Design review of the part built by this model. Coordinates are the model's own, in mm. Give positions to 0.01 mm unless a question says otherwise; leave off trailing zeros. Use CSV: the item, a comma, the result in double quotes.
```python
from build123d import *

# Parameters (mm, degrees)
SKETCH1_R               = 2.5
EXTRUDE1_DEPTH          = 510
CUT_EXTRUDE1_DEPTH      = 511.979451642
CUT_EXTRUDE1_DEPTH_BACK = 511.979451642
SKETCH2_W               = 3.3
SKETCH2_H               = 11.078679656


with BuildPart() as part:
    # Sketch1 → Extrude1 (new body)
    with BuildSketch(Plane.XY):
        with BuildLine():
            Line((0, 3.9), (-2.010912703, 3.9))
            ThreePointArc((-2.010912703, 3.9), (-2.776279568, 4.052240935), (-3.425126266, 4.485786438))
            Line((-3.425126266, 4.485786438), (-5.539339828, 6.6))
            Line((-5.539339828, 6.6), (-5.539339828, 8.2))
            Line((-5.539339828, 8.2), (-3.1, 8.2))
            Line((-3.1, 8.2), (-3.1, 9.5))
            Line((-3.1, 9.5), (-3.4, 9.5))
            ThreePointArc((-3.4, 9.5), (-3.541421356, 9.558578644), (-3.6, 9.7))
            Line((-3.6, 9.7), (-3.6, 10))
            Line((-3.6, 10), (-8.5, 10))
            Line((-8.5, 10), (-11.5, 10))
            Line((-11.5, 10), (-16.4, 10))
            Line((-16.4, 10), (-16.4, 9.7))
            ThreePointArc((-16.4, 9.7), (-16.458578644, 9.558578644), (-16.6, 9.5))
            Line((-16.6, 9.5), (-16.9, 9.5))
            Line((-16.9, 9.5), (-16.9, 8.2))
            Line((-16.9, 8.2), (-14.460660172, 8.2))
            Line((-14.460660172, 8.2), (-14.460660172, 6.6))
            Line((-14.460660172, 6.6), (-16.574873734, 4.485786438))
            ThreePointArc((-16.574873734, 4.485786438), (-17.223720432, 4.052240935), (-17.989087297, 3.9))
            Line((-17.989087297, 3.9), (-20, 3.9))
            Line((-20, 3.9), (-22.010912703, 3.9))
            ThreePointArc((-22.010912703, 3.9), (-22.776279568, 4.052240935), (-23.425126266, 4.485786438))
            Line((-23.425126266, 4.485786438), (-25.539339828, 6.6))
            Line((-25.539339828, 6.6), (-25.539339828, 8.2))
            Line((-25.539339828, 8.2), (-23.1, 8.2))
            Line((-23.1, 8.2), (-23.1, 9.5))
            Line((-23.1, 9.5), (-23.4, 9.5))
            ThreePointArc((-23.4, 9.5), (-23.541421356, 9.558578644), (-23.6, 9.7))
            Line((-23.6, 9.7), (-23.6, 10))
            Line((-23.6, 10), (-28.5, 10))
            ThreePointArc((-28.5, 10), (-29.560660172, 9.560660172), (-30, 8.5))
            Line((-30, 8.5), (-30, 3.6))
            Line((-30, 3.6), (-29.7, 3.6))
            ThreePointArc((-29.7, 3.6), (-29.558578644, 3.541421356), (-29.5, 3.4))
            Line((-29.5, 3.4), (-29.5, 3.1))
            Line((-29.5, 3.1), (-28.2, 3.1))
            Line((-28.2, 3.1), (-28.2, 5.539339828))
            Line((-28.2, 5.539339828), (-26.6, 5.539339828))
            Line((-26.6, 5.539339828), (-24.485786438, 3.425126266))
            ThreePointArc((-24.485786438, 3.425126266), (-24.052240935, 2.776279568), (-23.9, 2.010912703))
            Line((-23.9, 2.010912703), (-23.9, 0))
            Line((-23.9, 0), (-23.9, -2.010912703))
            ThreePointArc((-23.9, -2.010912703), (-24.052240935, -2.776279568), (-24.485786438, -3.425126266))
            Line((-24.485786438, -3.425126266), (-26.6, -5.539339828))
            Line((-26.6, -5.539339828), (-28.2, -5.539339828))
            Line((-28.2, -5.539339828), (-28.2, -3.1))
            Line((-28.2, -3.1), (-29.5, -3.1))
            Line((-29.5, -3.1), (-29.5, -3.4))
            ThreePointArc((-29.5, -3.4), (-29.558578644, -3.541421356), (-29.7, -3.6))
            Line((-29.7, -3.6), (-30, -3.6))
            Line((-30, -3.6), (-30, -8.5))
            ThreePointArc((-30, -8.5), (-29.560660172, -9.560660172), (-28.5, -10))
            Line((-28.5, -10), (-23.6, -10))
            Line((-23.6, -10), (-23.6, -9.7))
            ThreePointArc((-23.6, -9.7), (-23.541421356, -9.558578644), (-23.4, -9.5))
            Line((-23.4, -9.5), (-23.1, -9.5))
            Line((-23.1, -9.5), (-23.1, -8.2))
            Line((-23.1, -8.2), (-25.539339828, -8.2))
            Line((-25.539339828, -8.2), (-25.539339828, -6.6))
            Line((-25.539339828, -6.6), (-23.425126266, -4.485786438))
            ThreePointArc((-23.425126266, -4.485786438), (-22.776279568, -4.052240935), (-22.010912703, -3.9))
            Line((-22.010912703, -3.9), (-20, -3.9))
            Line((-20, -3.9), (-17.989087297, -3.9))
            ThreePointArc((-17.989087297, -3.9), (-17.223720432, -4.052240935), (-16.574873734, -4.485786438))
            Line((-16.574873734, -4.485786438), (-14.460660172, -6.6))
            Line((-14.460660172, -6.6), (-14.460660172, -8.2))
            Line((-14.460660172, -8.2), (-16.9, -8.2))
            Line((-16.9, -8.2), (-16.9, -9.5))
            Line((-16.9, -9.5), (-16.6, -9.5))
            ThreePointArc((-16.6, -9.5), (-16.458578644, -9.558578644), (-16.4, -9.7))
            Line((-16.4, -9.7), (-16.4, -10))
            Line((-16.4, -10), (-11.5, -10))
            Line((-11.5, -10), (-8.5, -10))
            Line((-8.5, -10), (-3.6, -10))
            Line((-3.6, -10), (-3.6, -9.7))
            ThreePointArc((-3.6, -9.7), (-3.541421356, -9.558578644), (-3.4, -9.5))
            Line((-3.4, -9.5), (-3.1, -9.5))
            Line((-3.1, -9.5), (-3.1, -8.2))
            Line((-3.1, -8.2), (-5.539339828, -8.2))
            Line((-5.539339828, -8.2), (-5.539339828, -6.6))
            Line((-5.539339828, -6.6), (-3.425126266, -4.485786438))
            ThreePointArc((-3.425126266, -4.485786438), (-2.776279568, -4.052240935), (-2.010912703, -3.9))
            Line((-2.010912703, -3.9), (0, -3.9))
            Line((0, -3.9), (2.010912703, -3.9))
            ThreePointArc((2.010912703, -3.9), (2.776279568, -4.052240935), (3.425126266, -4.485786438))
            Line((3.425126266, -4.485786438), (5.539339828, -6.6))
            Line((5.539339828, -6.6), (5.539339828, -8.2))
            Line((5.539339828, -8.2), (3.1, -8.2))
            Line((3.1, -8.2), (3.1, -9.5))
            Line((3.1, -9.5), (3.4, -9.5))
            ThreePointArc((3.4, -9.5), (3.541421356, -9.558578644), (3.6, -9.7))
            Line((3.6, -9.7), (3.6, -10))
            Line((3.6, -10), (8.5, -10))
            ThreePointArc((8.5, -10), (9.560660172, -9.560660172), (10, -8.5))
            Line((10, -8.5), (10, -3.6))
            Line((10, -3.6), (9.7, -3.6))
            ThreePointArc((9.7, -3.6), (9.558578644, -3.541421356), (9.5, -3.4))
            Line((9.5, -3.4), (9.5, -3.1))
            Line((9.5, -3.1), (8.2, -3.1))
            Line((8.2, -3.1), (8.2, -5.539339828))
            Line((8.2, -5.539339828), (6.6, -5.539339828))
            Line((6.6, -5.539339828), (4.485786438, -3.425126266))
            ThreePointArc((4.485786438, -3.425126266), (4.052240935, -2.776279568), (3.9, -2.010912703))
            Line((3.9, -2.010912703), (3.9, 0))
            Line((3.9, 0), (3.9, 2.010912703))
            ThreePointArc((3.9, 2.010912703), (4.052240935, 2.776279568), (4.485786438, 3.425126266))
            Line((4.485786438, 3.425126266), (6.6, 5.539339828))
            Line((6.6, 5.539339828), (8.2, 5.539339828))
            Line((8.2, 5.539339828), (8.2, 3.1))
            Line((8.2, 3.1), (9.5, 3.1))
            Line((9.5, 3.1), (9.5, 3.4))
            ThreePointArc((9.5, 3.4), (9.558578644, 3.541421356), (9.7, 3.6))
            Line((9.7, 3.6), (10, 3.6))
            Line((10, 3.6), (10, 8.5))
            ThreePointArc((10, 8.5), (9.560660172, 9.560660172), (8.5, 10))
            Line((8.5, 10), (3.6, 10))
            Line((3.6, 10), (3.6, 9.7))
            ThreePointArc((3.6, 9.7), (3.541421356, 9.558578644), (3.4, 9.5))
            Line((3.4, 9.5), (3.1, 9.5))
            Line((3.1, 9.5), (3.1, 8.2))
            Line((3.1, 8.2), (5.539339828, 8.2))
            Line((5.539339828, 8.2), (5.539339828, 6.6))
            Line((5.539339828, 6.6), (3.425126266, 4.485786438))
            ThreePointArc((3.425126266, 4.485786438), (2.776279568, 4.052240935), (2.010912703, 3.9))
            Line((2.010912703, 3.9), (0, 3.9))
        make_face()
        Circle(SKETCH1_R, mode=Mode.SUBTRACT)
        with Locations(Location((-20, 0, 0), (0, 0, 180))):
            Circle(SKETCH1_R, mode=Mode.SUBTRACT)
        with BuildLine():
            Line((-9.7, 3.6), (-10, 3.6))
            ThreePointArc((-10, 3.6), (-10.141421356, 3.541421356), (-10.2, 3.4))
            Line((-10.2, 3.4), (-10.2, 3.1))
            Line((-10.2, 3.1), (-11.5, 3.1))
            Line((-11.5, 3.1), (-11.5, 5.539339828))
            Line((-11.5, 5.539339828), (-13.1, 5.539339828))
            Line((-13.1, 5.539339828), (-15.214213562, 3.425126266))
            ThreePointArc((-15.214213562, 3.425126266), (-15.647759065, 2.776279568), (-15.8, 2.010912703))
            Line((-15.8, 2.010912703), (-15.8, 0))
            Line((-15.8, 0), (-15.8, -2.010912703))
            ThreePointArc((-15.8, -2.010912703), (-15.647759065, -2.776279568), (-15.214213562, -3.425126266))
            Line((-15.214213562, -3.425126266), (-13.1, -5.539339828))
            Line((-13.1, -5.539339828), (-11.5, -5.539339828))
            Line((-11.5, -5.539339828), (-11.5, -3.1))
            Line((-11.5, -3.1), (-10.2, -3.1))
            Line((-10.2, -3.1), (-10.2, -3.4))
            ThreePointArc((-10.2, -3.4), (-10.141421356, -3.541421356), (-10, -3.6))
            Line((-10, -3.6), (-9.7, -3.6))
            ThreePointArc((-9.7, -3.6), (-9.558578644, -3.541421356), (-9.5, -3.4))
            Line((-9.5, -3.4), (-9.5, -3.1))
            Line((-9.5, -3.1), (-8.2, -3.1))
            Line((-8.2, -3.1), (-8.2, -5.539339828))
            Line((-8.2, -5.539339828), (-6.6, -5.539339828))
            Line((-6.6, -5.539339828), (-4.485786438, -3.425126266))
            ThreePointArc((-4.485786438, -3.425126266), (-4.052240935, -2.776279568), (-3.9, -2.010912703))
            Line((-3.9, -2.010912703), (-3.9, 0))
            Line((-3.9, 0), (-3.9, 2.010912703))
            ThreePointArc((-3.9, 2.010912703), (-4.052240935, 2.776279568), (-4.485786438, 3.425126266))
            Line((-4.485786438, 3.425126266), (-6.6, 5.539339828))
            Line((-6.6, 5.539339828), (-8.2, 5.539339828))
            Line((-8.2, 5.539339828), (-8.2, 3.1))
            Line((-8.2, 3.1), (-9.5, 3.1))
            Line((-9.5, 3.1), (-9.5, 3.4))
            ThreePointArc((-9.5, 3.4), (-9.558578644, 3.541421356), (-9.7, 3.6))
        make_face(mode=Mode.SUBTRACT)
    extrude(amount=EXTRUDE1_DEPTH)

    # Sketch2 → Cut-Extrude1 (cut, two sides: drawn at the far end of the back side and taken through both)
    with BuildSketch(Plane.XY.offset(510).offset(-CUT_EXTRUDE1_DEPTH_BACK)):
        with Locations((-9.85, 0)):
            Rectangle(SKETCH2_W, SKETCH2_H)
    extrude(amount=CUT_EXTRUDE1_DEPTH + CUT_EXTRUDE1_DEPTH_BACK, mode=Mode.SUBTRACT)


solid = part.part
```
(1) For line 1 along X through (y, z) = (7.5, 488); line 2 along Y through (x, z) = (-25.5, 217); line 3 along X through (y, z) = (0.25, 37.5), list the stretches that pass through material, from the lowest coordinate up. Write a range as [from, to].
Established:
line 1,"x = [-30, -25.54], [-14.46, -5.54], [5.54, 10]"
line 2,"y = [-10, -8.2], [-6.56, -4.44], [4.44, 6.56], [8.2, 10]"
line 3,"x = [-23.9, -22.49], [-17.51, -15.8], [-3.9, -2.49], [2.49, 3.9]"
(2) Take a section at A-A (z = 417). State how many separate pieces and enclosed holes the cut face has, then the cut area to 3 significant figures.
Established:
separate pieces,"1"
enclosed holes,"3"
area,"331 mm2"
(3) Clearance check with flat-ended pins moving along their axes: pin 1 (2 mm diameter, centred on x = 2, z = 161, fed in from -Y); pin 2 (4.5 mm diameter, centred on y = 0.5, z = 344, fed in from -X); pin 3 (2 mm diameter, centred on x = -20, z = 357, fed in from -Y). State where each tip first meets the part, or that it passes through.
Established:
pin 1,"stops at y = -4.16"
pin 2,"stops at x = -24.04"
pin 3,"stops at y = -3.9"
